Input: dimensioned drawing with shaded views. Units: mm. Origin: part minimum x, y, z. Coordinates: 2 decimals unless noted, no trailing zeros. Order: outer loops, then holes, each group sorted by start corner. A loop starts at its lowest first (then second) coordinate and runs counter-clockwise, first axis right, second up. Notation, with made-up numbers: (17.25, -10.75) -> (58.25, -10.75) arc R23 cw to (58.25, -1.75) -> close; hole circle Ø2 at (15.25, 61.5). An arc over 180 degrees is marked (long way). Answer in a Markdown table with one row per item. Add a question column.
1) Section query C-C on x = 0.6. Return the cut outline in (y, z).
2) Contact query for flat-ended pins moving along their axis: P1, Ø6, axis at y = 12.5, z = 62.5, coming from the -X side; P2, Ø1, axis at x = 0.5, y = 4.5, coming from the +Z side. Output: stop coordinate, or through.
3) Section query B-B on z = 15. Return the cut outline in (x, y), then the cut area to 3 significant figures.
4) Section query A-A on y = 12.5. Return the cut outline in (x, z), then the cut area to 3 significant figures.
5) Section query D-D on y = 8.5. Return the cut outline in (x, z), then the cut area to 3 significant figures.
6) Ray query, line 1 (Z direction, x = 2.1, y = 12.5); line 2 (Z direction, x = 2.8, y = 9.5); line 3 (Y direction, x = 2.3, z = 62). Return the intervals inside material, ascending. Write a range as from..to.
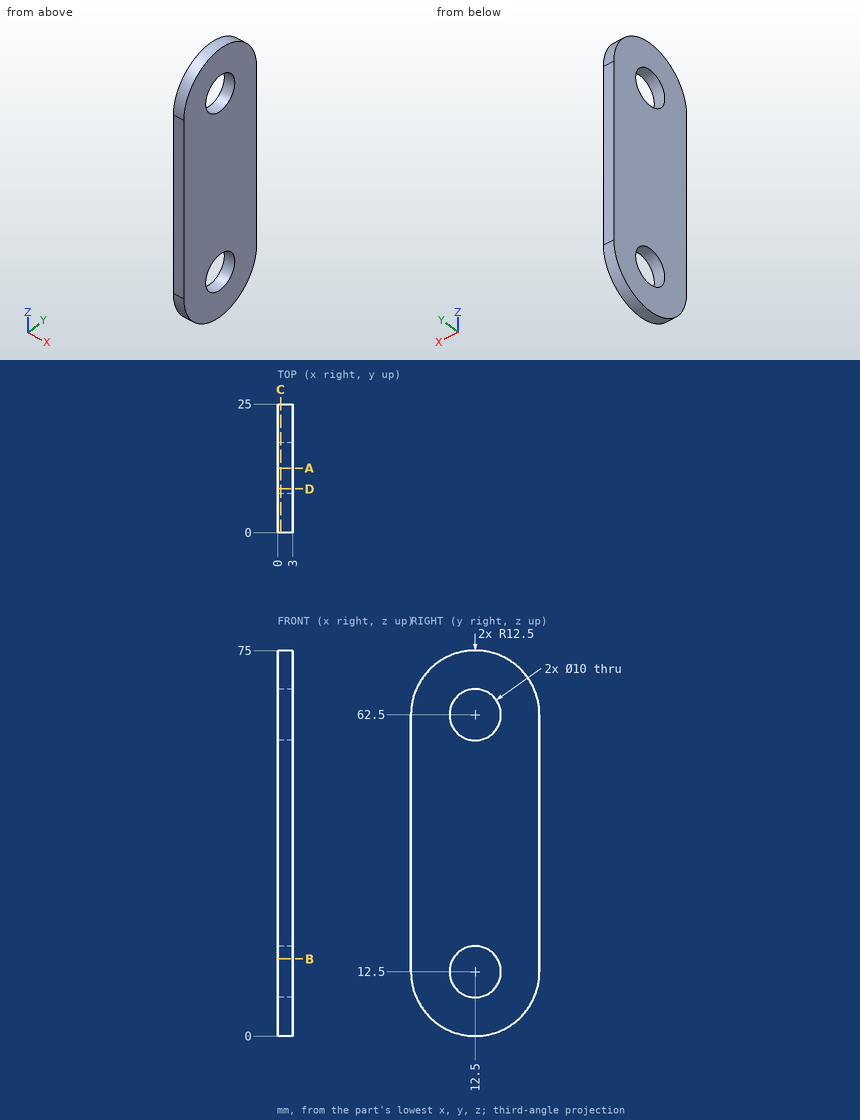
Result:
| question | item | result |
|---|---|---|
| 1 | outline | (0, 12.5) arc R12.5 ccw to (25, 12.5) -> (25, 62.5) arc R12.5 ccw to (0, 62.5) -> close; hole circle Ø10 at (12.5, 12.5); hole circle Ø10 at (12.5, 62.5) |
| 2 | P1 | through |
| 2 | P2 | z = 72.5 |
| 3 | outline | (0, 0) -> (3, 0) -> (3, 8.17) -> (0, 8.17) -> close; (0, 16.83) -> (3, 16.83) -> (3, 25) -> (0, 25) -> close |
| 3 | area | 49.0 mm2 |
| 4 | outline | (0, 0) -> (3, 0) -> (3, 7.5) -> (0, 7.5) -> close; (0, 17.5) -> (3, 17.5) -> (3, 57.5) -> (0, 57.5) -> close; (0, 67.5) -> (3, 67.5) -> (3, 75) -> (0, 75) -> close |
| 4 | area | 165 mm2 |
| 5 | outline | (0, 0.66) -> (3, 0.66) -> (3, 9.5) -> (0, 9.5) -> close; (0, 15.5) -> (3, 15.5) -> (3, 59.5) -> (0, 59.5) -> close; (0, 65.5) -> (3, 65.5) -> (3, 74.34) -> (0, 74.34) -> close |
| 5 | area | 185 mm2 |
| 6 | line 1 | 0..7.5, 17.5..57.5, 67.5..75 |
| 6 | line 2 | 0.37..8.5, 16.5..58.5, 66.5..74.63 |
| 6 | line 3 | 0..7.53, 17.47..25 |
